```python
from build123d import *

# Parameters (mm, degrees)
BOSS_EXTRUDE1_DEPTH = 5.96
CUT_EXTRUDE1_REACH  = 10.869
SKETCH2_R           = 2


with BuildPart() as part:
    # Sketch1 → Boss-Extrude1 (new body)
    with BuildSketch(Plane(origin=(0, 0, 0), x_dir=(0, 1, 0), z_dir=(0, 0, 1))):
        Polygon((4.965212315, 0), (2.482606158, 4.3), (-2.482606158, 4.3), (-4.965212315, 0), (-2.482606158, -4.3), (2.482606158, -4.3), align=None)
    extrude(amount=BOSS_EXTRUDE1_DEPTH)

    # Sketch2 → Cut-Extrude1 (cut, up to next)
    with BuildSketch(Plane(origin=(0, 0, 0), x_dir=(0, 1, 0), z_dir=(0, 0, 1)), mode=Mode.PRIVATE) as cut_extrude1_sk1:
        with Locations(Location((0, 0, 0), (0, 0, 270))):
            Circle(SKETCH2_R)
    cut_extrude1_tool1 = extrude(cut_extrude1_sk1.sketch, amount=CUT_EXTRUDE1_REACH, mode=Mode.PRIVATE) & part.part
    add(cut_extrude1_tool1.solids().sort_by_distance((0, 0, 0))[0], mode=Mode.SUBTRACT)


solid = part.part
```
Build history of the part. All positions in model axes, mm. Coordinates: 2 decimals unless noted, no trailing zeros. Order: outer loops, then holes, each group sorted by start corner. A loop starts at its lowest first (then second) coordinate and runs counter-clockwise, first axis right, second up. Notation, with made-up numbers: (58.5, 18.25) -> (97.5, 18.25) arc R20 ccw to (97.5, 33.25) -> close; hole circle Ø5 at (20.25, 87.25). An arc over 180 degrees is marked (long way). Answer in a Markdown table with one row per item. Add a question column.
Q1. Drop flat-ended pins along their axis: pin 1 (3 mm diameter, centred on x = 3.5, z = 1.5, fed in from -Y); pin 2 (4.5 mm diameter, centred on x = 0, y = 0, fed in from -Z). Give the stop position or say it passes through.
Q2. Wall check: line 1 along X through (y, z) = (0, 3.75); line 2 along Y through (x, z) = (-0.5, 1.6); line 3 along Y through (x, z) = (-1, 4.75). Give the ranges that are in metal, low to high. Write a range as [from, to].
Q3. Band-saw the part on A-A, the plane z = 4.4. List the corners of the cut face in (x, y), then the cut area to 3 significant figures.
Q4. Mould opens along Y. For faces 1 (the face through (-2.18, -3.707, 2.938)), 2 (the face through (4.3, 0, 3)), 3 (the face through (0, -2, 3)) say: +Y half, -Y half, draft (parallel to the pull), parting line (faces both ways), or undercut.
Q5. Band-saw the part on B-B, the plane y = -1.75. List the corners of the cut face in (x, z), then the cut area to 3 significant figures.
Q6. Band-saw the part on C-C, the plane x = -1.5. List the corners of the cut face in (y, z).
Q7. Band-saw the part on D-D, the plane y = -2.75. List the corners of the cut face in (x, z).
Answers follow:
| question | item | result |
|---|---|---|
| 1 | pin 1 | y = -3.81 |
| 1 | pin 2 | z = 0 |
| 2 | line 1 | [-4.3, -2], [2, 4.3] |
| 2 | line 2 | [-4.68, -1.94], [1.94, 4.68] |
| 2 | line 3 | [-4.39, -1.73], [1.73, 4.39] |
| 3 | outline | (-4.3, -2.48) -> (0, -4.97) -> (4.3, -2.48) -> (4.3, 2.48) -> (0, 4.97) -> (-4.3, 2.48) -> close; hole circle Ø4 at (0, 0) |
| 3 | area | 51.5 mm^2 |
| 4 | face 1 | -Y half |
| 4 | face 2 | draft |
| 4 | face 3 | undercut |
| 5 | outline | (-4.3, 0) -> (-0.97, 0) -> (-0.97, 5.96) -> (-4.3, 5.96) -> close; (0.97, 0) -> (4.3, 0) -> (4.3, 5.96) -> (0.97, 5.96) -> close |
| 5 | area | 39.7 mm^2 |
| 6 | outline | (-4.1, 0) -> (-1.32, 0) -> (-1.32, 5.96) -> (-4.1, 5.96) -> close; (1.32, 0) -> (4.1, 0) -> (4.1, 5.96) -> (1.32, 5.96) -> close |
| 7 | outline | (-3.84, 0) -> (3.84, 0) -> (3.84, 5.96) -> (-3.84, 5.96) -> close |
